Autodesk Inventor part; units mm, degrees
ref_plane "YZ Plane" through (0, 0, 0) normal (1, 0, 0) x (0, 1, 0)
ref_plane "XZ Plane" through (0, 0, 0) normal (0, 1, 0) x (-1, 0, 0)
ref_plane "XY Plane" through (0, 0, 0) normal (0, 0, 1) x (1, 0, 0)
sketch "Sketch1" plane through (0, 0, 0) normal (0, 0, 1) x (1, 0, 0)
  circle A0 centre (35.3094, -51.3621) radius 1.985
  circle A1 centre (-35.3094, -51.3621) radius 1.985
  circle A2 centre (-35.3094, 51.3621) radius 1.985
  circle A3 centre (35.3094, 51.3621) radius 1.985
  line L0 (28.5119, 50.05) -> (-28.5119, 50.05)
  arc A4 (-28.5119, 50.05) -> (-29.6663, 51.7567) centre (-32.2906, 48.7379) ccw
  line L1 (-32.6852, 54.381) -> (-29.6663, 51.7567)
  arc A5 (-32.6852, 54.381) -> (-37.9337, 48.3433) centre (-35.3094, 51.3621) ccw
  line L2 (-33.8, 44.7499) -> (-37.9337, 48.3433)
  line L3 (-33.8, 44.7499) -> (-33.8, -44.7499)
  line L4 (-37.9337, -48.3433) -> (-33.8, -44.7499)
  arc A6 (-37.9337, -48.3433) -> (-32.6852, -54.381) centre (-35.3094, -51.3621) ccw
  line L5 (-29.6663, -51.7567) -> (-32.6852, -54.381)
  arc A7 (-29.6663, -51.7567) -> (-28.5119, -50.05) centre (-32.2906, -48.7379) ccw
  line L6 (-28.5119, -50.05) -> (28.5119, -50.05)
  arc A8 (28.5119, -50.05) -> (29.6663, -51.7567) centre (32.2906, -48.7379) ccw
  line L7 (32.6852, -54.381) -> (29.6663, -51.7567)
  arc A9 (32.6852, -54.381) -> (37.9337, -48.3433) centre (35.3094, -51.3621) ccw
  line L8 (33.8, -44.7499) -> (37.9337, -48.3433)
  line L9 (33.8, -44.7499) -> (33.8, 44.7499)
  line L10 (37.9337, 48.3433) -> (33.8, 44.7499)
  arc A10 (37.9337, 48.3433) -> (32.6852, 54.381) centre (35.3094, 51.3621) ccw
  line L11 (29.6663, 51.7567) -> (32.6852, 54.381)
  arc A11 (29.6663, 51.7567) -> (28.5119, 50.05) centre (32.2906, 48.7379) ccw
  line L12 (-30.6, -44.85) -> (-30.6, 44.85)
  arc A12 (-28.6, 46.85) -> (-30.6, 44.85) centre (-28.6, 44.85) ccw
  line L13 (-28.6, 46.85) -> (28.6, 46.85)
  arc A13 (30.6, 44.85) -> (28.6, 46.85) centre (28.6, 44.85) ccw
  line L14 (30.6, 44.85) -> (30.6, -44.85)
  arc A14 (28.6, -46.85) -> (30.6, -44.85) centre (28.6, -44.85) ccw
  line L15 (28.6, -46.85) -> (-28.6, -46.85)
  arc A15 (-30.6, -44.85) -> (-28.6, -46.85) centre (-28.6, -44.85) ccw
  point P0 (0, 0)
extrude "Extrusion1" add sketch "Sketch1" along normal blind 2 contours A11 L11 A10 L10 L9 L8 A9 L7 A8 L6 A7 L5 A6 L4 L3 L2 A5 L1 A4 L0 | L12 A12 L13 A13 L14 A14 L15 A15
sketch "Sketch3" plane through (0, 0, 2) normal (0, 0, 1) x (1, 0, 0)
  line L0 (-5.7986, 18.4674) -> (8.3133, 18.4674)
  line L1 (8.3133, 18.4674) -> (8.3133, 4.4942)
  line L2 (8.3133, 4.4942) -> (-5.7986, 4.4942)
  line L3 (-5.7986, 4.4942) -> (-5.7986, 18.4674)
  line L4 (-8.1427, -5.5192) -> (-8.1427, 28.4808) construction
  line L5 (-6.1427, -5.5192) -> (-6.1427, 28.4808)
  line L6 (-10.1427, 28.4808) -> (-10.1427, -5.5192)
  arc A0 (-10.1427, -5.5192) -> (-6.1427, -5.5192) centre (-8.1427, -5.5192) ccw
  arc A1 (-6.1427, 28.4808) -> (-10.1427, 28.4808) centre (-8.1427, 28.4808) ccw
  arc A2 (-0.1427, 28.4808) -> (-4.1427, 28.4808) centre (-2.1427, 28.4808) ccw
  line L7 (-0.1427, -5.5192) -> (-0.1427, 28.4808)
  line L8 (-4.1427, 28.4808) -> (-4.1427, -5.5192)
  arc A3 (-4.1427, -5.5192) -> (-0.1427, -5.5192) centre (-2.1427, -5.5192) ccw
  line L9 (5.8573, -5.5192) -> (5.8573, 28.4808)
  arc A4 (5.8573, 28.4808) -> (1.8573, 28.4808) centre (3.8573, 28.4808) ccw
  line L10 (1.8573, 28.4808) -> (1.8573, -5.5192)
  arc A5 (1.8573, -5.5192) -> (5.8573, -5.5192) centre (3.8573, -5.5192) ccw
  line L11 (-16.1427, 28.4808) -> (-16.1427, -5.5192)
  arc A6 (-12.1427, 28.4808) -> (-16.1427, 28.4808) centre (-14.1427, 28.4808) ccw
  line L12 (-12.1427, -5.5192) -> (-12.1427, 28.4808)
  arc A7 (-16.1427, -5.5192) -> (-12.1427, -5.5192) centre (-14.1427, -5.5192) ccw
  line L13 (-22.1427, 28.4808) -> (-22.1427, -5.5192)
  arc A8 (-18.1427, 28.4808) -> (-22.1427, 28.4808) centre (-20.1427, 28.4808) ccw
  line L14 (-18.1427, -5.5192) -> (-18.1427, 28.4808)
  arc A9 (-22.1427, -5.5192) -> (-18.1427, -5.5192) centre (-20.1427, -5.5192) ccw
  point P0 (0, 0)
  point P1 (-8.1427, 11.4808)
  dimension "d8" = 17
  dimension "d9" = 4
  dimension "d12" = 6
  dimension "d19" = 6
  dimension "d26" = 6
extrude "Extrusion3" cut sketch "Sketch3" against normal up to surface (2 mm away) contours L8 A2 L7 L0 | L0 L7 L2 L8 | L2 L7 A3 L8 | L10 A4 L9 L0 | L0 L9 L2 L10 | L2 L9 A5 L10 | A0 L6 A1 L5 | A6 L12 A7 L11 | A8 L14 A9 L13
properties part number "Case Cover Rev D"
Can you work these out from the model? Positions are in its coordinate system, mm. A direction names the side the tool comes from. Round coordinates to 2 decimals unless told otherwise and drop trailing zeros. Loops run counter-clockwise (first coordinate to the right, second up) from the corner with the lowest first, then second, coordinate; pieces in that order, holes last. Notation, with made-up numbers: (55, -20.5) - (83, -20.5) arc R25 ccw to (83, -6.5) - close; hole circle Ø4 at (-12, -7). An arc over 180 degrees is marked (long way). Write item = value, one per line. Start each with the question number.
(1) If I drill on probe 1 along X at (y, z) = (0, 0.95); probe 2 along X at (y, z) = (-6, 1.65); probe 3 along Y at (x, z) = (35, 0.55), over which ranges is the centre line in solid material (lowest first)? Write a range as [from, to].
(2) If we section it at C-C (x = 16.5): Please give me the cut outline in (y, z), and give its area (3 significant figures).
(3) If we section it at B-B (x = -14): Please give me the cut outline in (y, z).
(4) For P1, Ø0.6, axis at y = 11, z = 1, coming from the +X side; P2, Ø1, axis at y = 10.5, z = 1, coming from the -X side; P3, Ø3, axis at x = -35.31, y = -51.36, coming from the +Z side (3 decimals), each with a flat end and sliding along its axis, tell me the tip position at first contact or that it passes through.
(5) If we mould it in two halves opening along X, with no side actions, what happens to faces 1 (the face through (31.2, -53.09, 0.99)), 2 (the face through (8, 1, 2)), 3 (the face through (-33.416, 50.766, 0.986)), 4 (the face through (35.838, -46.521, 0.986))? For each: released by +X, released by -X, zero draft, split by the parting line, or undercut.
(6) If we section it at D-D (y = 37.5): Please give me the cut outline in (x, z).
(7) For faces 5 (the face through (-35.896, -46.572, 0.986)), 6 (the face through (-31.155, -53.05, 0.986)), 7 (the face through (31.155, 53.05, 0.986)), 8 (the face through (35.896, 46.572, 0.986)), which set-ups out of +Z, -Z, +X, -X, +Y, -Y let a thin tool reach every point of the face, with its end or its side?
(8) If we section it at A-A (y = 12.5): Please give me the cut outline in (x, z), and give its area (3 significant figures).
Ans:
q1.probe_1 = [-33.8, -22.14], [-18.14, -16.14], [-12.14, -10.14], [-6.14, -4.14], [-0.14, 1.86], [5.86, 33.8]
q1.probe_2 = [-33.8, -22.08], [-18.2, -16.08], [-12.2, -10.08], [-6.2, -4.08], [-0.2, 1.92], [5.8, 33.8]
q1.probe_3 = [-55.35, -53.32], [-49.4, -45.79], [45.79, 49.4], [53.32, 55.35]
q2.outline = (-50.05, 0) - (50.05, 0) - (50.05, 2) - (-50.05, 2) - close
q2.area = 200 mm²
q3.outline = (-50.05, 0) - (-7.51, 0) - (-7.51, 2) - (-50.05, 2) - close; (30.48, 0) - (50.05, 0) - (50.05, 2) - (30.48, 2) - close
q4.P1 = 33.8
q4.P2 = -33.8
q4.P3 = through
q5.face_1 = undercut
q5.face_2 = zero draft
q5.face_3 = undercut
q5.face_4 = released by +X
q6.outline = (-33.8, 0) - (33.8, 0) - (33.8, 2) - (-33.8, 2) - close
q7.face_5 = +Z, -Z, -X
q7.face_6 = +Z, -Z, -Y
q7.face_7 = +Z, -Z, +Y
q7.face_8 = +Z, -Z, +X
q8.outline = (-33.8, 0) - (-22.14, 0) - (-22.14, 2) - (-33.8, 2) - close; (-18.14, 0) - (-16.14, 0) - (-16.14, 2) - (-18.14, 2) - close; (-12.14, 0) - (-10.14, 0) - (-10.14, 2) - (-12.14, 2) - close; (-6.14, 0) - (-4.14, 0) - (-4.14, 2) - (-6.14, 2) - close; (-0.14, 0) - (1.86, 0) - (1.86, 2) - (-0.14, 2) - close; (5.86, 0) - (33.8, 0) - (33.8, 2) - (5.86, 2) - close
q8.area = 95.2 mm²
